Design review of the part shown in the three views and the two pictorial views. Dimensions are in mm from the part's minimum x, y and z. Coordinates: 2 decimals unless noted, no trailing zeros. Write each loop counter-clockwise with the first axis right and the second up, starting at its lowest first coordinate (ties: lowest second). Pieces come first, ordered by that corner, then holes. Notation, with made-up numbers: (-17, -34) - (-6, -34) arc R34 cw to (-6, 4) - close; hole circle Ø11 at (-13.75, -20). An arc over 180 degrees is marked (long way). Write each question's results on one line, items separated by ' | '.
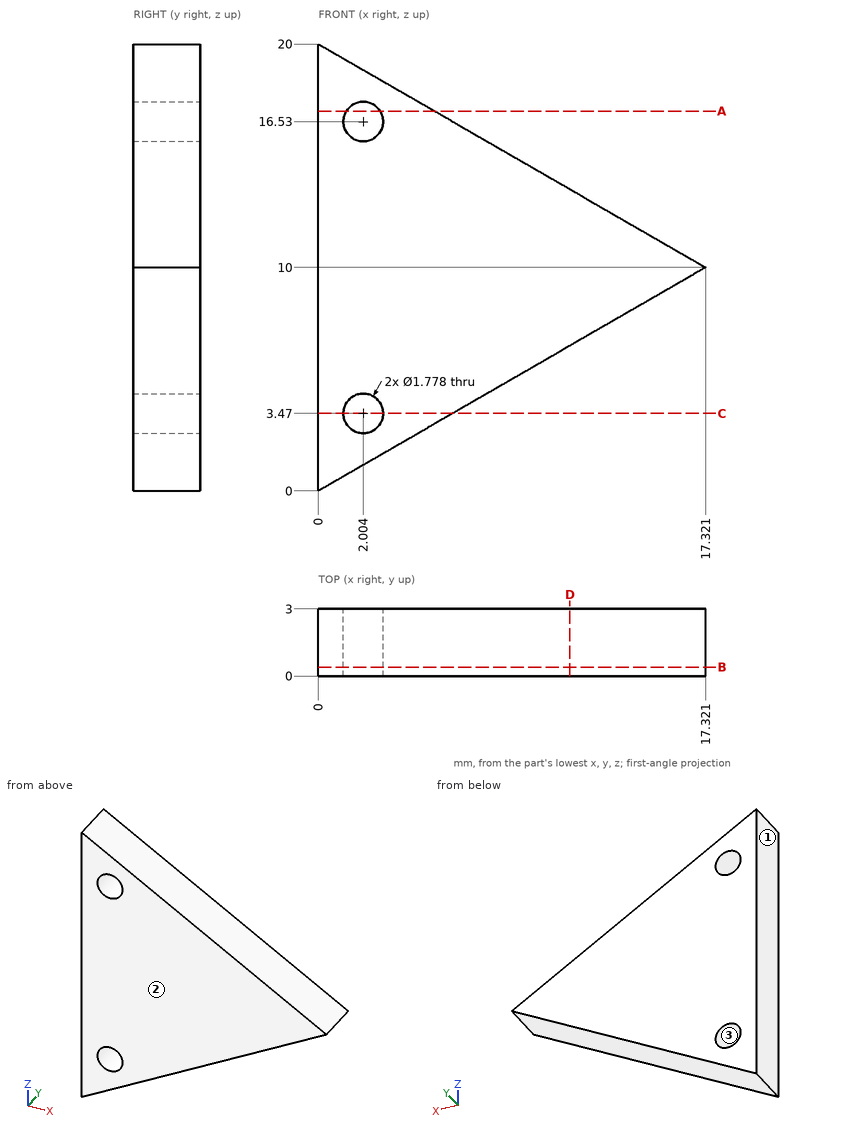
Q1. Take a section at B-B on y = 0.4. State the section outline as (x, z) points.
Results found:
outline: (0, 0) - (17.32, 10) - (0, 20) - close; hole circle Ø1.78 at (2, 3.47); hole circle Ø1.78 at (2, 16.53)
Q2. Take a section at C-C on z = 3.47. State the section outline as (x, y) points (1 decimal), plus the area to 3 significant figures.
Results found:
outline: (0, 0) - (1.1, 0) - (1.1, 3) - (0, 3) - close; (2.9, 0) - (6, 0) - (6, 3) - (2.9, 3) - close | area: 12.7 mm2
Q3. For pin 1 (1.4 mm diameter, centred on x = 2, z = 3.47, fed in from +Y); pin 2 (1 mm diameter, centred on y = 1, z = 15, fed in from -X), all flat-tipped, find the tip position at first contact; note any pin that passes through.
Results found:
pin 1: through | pin 2: x = 0
Q4. Take a section at A-A on z = 17. State the section outline as (x, y) points.
Results found:
outline: (0, 0) - (1.25, 0) - (1.25, 3) - (0, 3) - close; (2.76, 0) - (5.2, 0) - (5.2, 3) - (2.76, 3) - close
Q5. Take a section at D-D on x = 11.25. State the section outline as (y, z) points (1 decimal), plus the area to 3 significant figures.
Results found:
outline: (0, 6.5) - (3, 6.5) - (3, 13.5) - (0, 13.5) - close | area: 21.0 mm2
Q6. Wall thickness on line 1 along Z through (x, y) = (2.25, 2.4) (1 decimal); line 2 along X through (y, z) = (2.85, 16) (1 decimal); line 3 along X through (y, z) = (0.75, 16.53) (1 decimal): over which ranges is each line inside the solid? List them lowest first. Write a range as from..to.
Results found:
line 1: 1.3..2.6, 4.3..15.7, 17.4..18.7 | line 2: 0..1.3, 2.7..6.9 | line 3: 0..1.1, 2.9..6
Q7. Mouldability with a two-part tool opening along X and no side actions: class the marked faces 1, 2 and 3 as pulls with the +X half, pulls with the -X half, needs draft (parallel to the pull), parting line crosses it, or undercut.
Results found:
face 1: pulls with the -X half | face 2: needs draft | face 3: undercut
